from build123d import *

# Parameters (mm, degrees)
F1_DEPTH = 2
F2_R     = 1.27
F3_D     = 2.5908
F3_DEPTH = 3.81
F3_TIP   = 0.7783548459


with BuildPart() as f1:
    # F0 (on Top) → F1 (new body)
    with BuildSketch(Plane.XY):
        with BuildLine():
            Line((22.5, -20.12), (22.5, -12.5))
            Line((22.5, -12.5), (12.975, -12.5))
            Line((12.975, -12.5), (12.975, -13.77))
            ThreePointArc((12.975, -13.77), (14.7710512242, -14.5139487758), (15.515, -16.31))
            ThreePointArc((15.515, -16.31), (14.7710512242, -18.1060512242), (12.975, -18.85))
            Line((12.975, -18.85), (12.975, -20.12))
            Line((12.975, -20.12), (22.5, -20.12))
        make_face()
        with BuildLine():
            Line((12.975, -12.5), (22.5, -12.5))
            Line((22.5, -12.5), (22.5, 0))
            Line((22.5, 0), (20.975, 0))
            ThreePointArc((20.975, 0), (18.6318542495, -5.6568542495), (12.975, -8))
            Line((12.975, -8), (12.975, -12.5))
        make_face()
        with BuildLine():
            Line((12.975, -13.77), (12.975, -12.5))
            Line((12.975, -12.5), (-22.5, -12.5))
            Line((-22.5, -12.5), (-22.5, -16.31))
            Line((-22.5, -16.31), (-12.54, -16.31))
            ThreePointArc((-12.54, -16.31), (-10, -13.77), (-7.46, -16.31))
            Line((-7.46, -16.31), (10.435, -16.31))
            ThreePointArc((10.435, -16.31), (11.1789487758, -14.5139487758), (12.975, -13.77))
        make_face()
        with BuildLine():
            Line((-22.5, -12.5), (12.975, -12.5))
            Line((12.975, -12.5), (12.975, -8))
            ThreePointArc((12.975, -8), (4.975, 0), (12.975, 8))
            ThreePointArc((12.975, 8), (18.6318542495, 5.6568542495), (20.975, 0))
            Line((20.975, 0), (22.5, 0))
            Line((22.5, 0), (22.5, 12.5))
            Line((22.5, 12.5), (-22.5, 12.5))
            Line((-22.5, 12.5), (-22.5, 0))
            Line((-22.5, 0), (-22.5, -12.5))
        make_face()
        Polygon((-20, -10), (-20, 0), (-20, 10), (-10, 10), (0, 10), (0, 0), (0, -10), (-10, -10), align=None, mode=Mode.SUBTRACT)
        with BuildLine():
            Line((-22.5, -20.12), (12.975, -20.12))
            Line((12.975, -20.12), (12.975, -18.85))
            ThreePointArc((12.975, -18.85), (11.1789487758, -18.1060512242), (10.435, -16.31))
            Line((10.435, -16.31), (-7.46, -16.31))
            ThreePointArc((-7.46, -16.31), (-10, -18.85), (-12.54, -16.31))
            Line((-12.54, -16.31), (-22.5, -16.31))
            Line((-22.5, -16.31), (-22.5, -20.12))
        make_face()
        with BuildLine():
            ThreePointArc((12.975, 8), (4.975, 0), (12.975, -8))
            Line((12.975, -8), (12.975, -4))
            ThreePointArc((12.975, -4), (8.975, 0), (12.975, 4))
            Line((12.975, 4), (12.975, 8))
        make_face()
        with BuildLine():
            Line((16.975, 0), (20.975, 0))
            ThreePointArc((20.975, 0), (18.6318542495, 5.6568542495), (12.975, 8))
            Line((12.975, 8), (12.975, 4))
            ThreePointArc((12.975, 4), (15.8034271247, 2.8284271247), (16.975, 0))
        make_face()
        with BuildLine():
            Line((12.975, -4), (12.975, -8))
            ThreePointArc((12.975, -8), (18.6318542495, -5.6568542495), (20.975, 0))
            Line((20.975, 0), (16.975, 0))
            ThreePointArc((16.975, 0), (15.8034271247, -2.8284271247), (12.975, -4))
        make_face()
        with BuildLine():
            ThreePointArc((0, 0), (-2.9289321881, -7.0710678119), (-10, -10))
            Line((-10, -10), (0, -10))
            Line((0, -10), (0, 0))
        make_face()
        with BuildLine():
            ThreePointArc((-10, -10), (-17.0710678119, -7.0710678119), (-20, 0))
            Line((-20, 0), (-20, -10))
            Line((-20, -10), (-10, -10))
        make_face()
        with BuildLine():
            Line((-20, 10), (-20, 0))
            ThreePointArc((-20, 0), (-17.0710678119, 7.0710678119), (-10, 10))
            Line((-10, 10), (-20, 10))
        make_face()
        with BuildLine():
            Line((0, 10), (-10, 10))
            ThreePointArc((-10, 10), (-2.9289321881, 7.0710678119), (0, 0))
            Line((0, 0), (0, 10))
        make_face()
    extrude(amount=F1_DEPTH)

    # F2
    f2_edges = [f1.edges().sort_by_distance(p)[0] for p in [
        (-22.5, 12.5, 1),
        (22.5, 12.5, 1),
        (-22.5, -20.12, 1),
        (22.5, -20.12, 1),
    ]]
    fillet(f2_edges, radius=F2_R)

    # F3
    with Locations(Plane(origin=(0, 0, 0), x_dir=(1, 0, 0), z_dir=(0, 0, -1))):
        with Locations((-20, -10), (0, -10), (0, 10), (-20, 10), (12.975, -8), (12.975, 8)):
            Hole(F3_D / 2, depth=F3_DEPTH)
            with Locations((0, 0, -(F3_DEPTH + F3_TIP / 2))):  # 118° drill point
                Cone(0, F3_D / 2, F3_TIP, mode=Mode.SUBTRACT)


solid = f1.part
Design review of the part built by this model. Coordinates are the model's own, in mm. Coordinates: 2 decimals unless noted, no trailing zeros. Order: outer loops, then holes, each group sorted by start corner. A loop starts at its lowest first (then second) coordinate and runs counter-clockwise, first axis right, second up. Notation, with made-up numbers: (5, -22.75) -> (62, -22.75) arc R13 cw to (62, -15.75) -> close; hole circle Ø6 at (-17.5, -34). An arc over 180 degrees is marked (long way). Use one line per item in the form item = value. Start each with the question number.
(1) Add section A-A on y = -8. State the section outline as (x, z) points, plus the area to 3 significant figures.
(2) Add section D-D on x = 11. State the section outline as (y, z) points, plus the area to 3 significant figures.
(3) The part is to be moulded in two halves that separate along Y. For faces 1 (the flat face through (0, 12.5, 1)), 2 (the flat face through (5, -4, 2)), 3 (the cylindrical face through (14.27, 7.94, 1.01)), say which applies: +Y half, -Y half, draft (parallel to the pull), parting line (faces both ways), or undercut.
(4) Insertion check: pin 1 (2.5 mm diameter, centred on x = -20, y = 10, fed in from -Z). The pin has a flat end and moves straight along its axis. Give the tip position at first contact, or say it passes through.
(5) Add section C-C on z = 1.65. Give the number of separate pieces and of enclosed holes in the cut face, plus the area to 3 significant figures.
(6) Add section B-B on x = -17.5. State the section outline as (y, z) points.
(7) For probe 1 along Y at (x, z) = (-10, 0.45); probe 2 along X at (y, z) = (-16.31, 0.4) (3 decimals); probe 3 along X at (y, z) = (-3.5, 1.95), list the stretches that pass through material, from the lowest coordinate up.
Answer block:
q1.outline = (-22.5, 0) -> (-16, 0) -> (-16, 2) -> (-22.5, 2) -> close; (-4, 0) -> (11.68, 0) -> (11.68, 2) -> (-4, 2) -> close; (14.27, 0) -> (22.5, 0) -> (22.5, 2) -> (14.27, 2) -> close
q1.area = 60.8 mm²
q2.outline = (-20.12, 0) -> (-17.91, 0) -> (-17.91, 2) -> (-20.12, 2) -> close; (-14.71, 0) -> (-3.48, 0) -> (-3.48, 2) -> (-14.71, 2) -> close; (3.48, 0) -> (12.5, 0) -> (12.5, 2) -> (3.48, 2) -> close
q2.area = 44.9 mm²
q3.face_1 = +Y half
q3.face_2 = draft
q3.face_3 = undercut
q4.pin_1 = through
q5.separate_pieces = 1
q5.enclosed_holes = 10
q5.area = 1,030 mm²
q6.outline = (-20.12, 0) -> (-6.61, 0) -> (-6.61, 2) -> (-20.12, 2) -> close; (6.61, 0) -> (12.5, 0) -> (12.5, 2) -> (6.61, 2) -> close
q7.probe_1 = -20.12 to -18.85, -13.77 to -10, 10 to 12.5
q7.probe_2 = -22.5 to -12.54, -7.46 to 10.435, 15.515 to 22.5
q7.probe_3 = -22.5 to -19.37, -0.63 to 11.04, 14.91 to 22.5
